from build123d import *

# Parameters (mm, degrees)
MODEL_R                 = 1.5
SALIENTE_EXTRUIR1_DEPTH = 3


with BuildPart() as part:
    # Model → Saliente-Extruir1 (new body)
    with BuildSketch(Plane.XY):
        with BuildLine():
            Line((149.34213351, 211.823953209), (158.34213351, 211.823953209))
            ThreePointArc((158.34213351, 211.823953209), (161.524114025, 210.505933724), (162.84213351, 207.323953209))
            Line((162.84213351, 207.323953209), (162.84213351, 193.823953209))
            Line((162.84213351, 193.823953209), (153.84213351, 193.823953209))
            Line((153.84213351, 193.823953209), (153.84213351, 202.823953209))
            Line((153.84213351, 202.823953209), (149.34213351, 202.823953209))
            ThreePointArc((149.34213351, 202.823953209), (144.84213351, 207.323953209), (149.34213351, 211.823953209))
        make_face()
        with Locations((149.34213351, 207.323953209)):
            Circle(MODEL_R, mode=Mode.SUBTRACT)
        with Locations((158.34213351, 207.323953209)):
            Circle(MODEL_R, mode=Mode.SUBTRACT)
        with BuildLine():
            Line((160.84213351, 196.698953209), (155.84213351, 196.698953209))
            ThreePointArc((155.84213351, 196.698953209), (155.311803424, 196.918623123), (155.09213351, 197.448953209))
            Line((155.09213351, 197.448953209), (155.09213351, 199.198953209))
            ThreePointArc((155.09213351, 199.198953209), (155.311803424, 199.729283295), (155.84213351, 199.948953209))
            Line((155.84213351, 199.948953209), (160.84213351, 199.948953209))
            ThreePointArc((160.84213351, 199.948953209), (161.372463595, 199.729283295), (161.59213351, 199.198953209))
            Line((161.59213351, 199.198953209), (161.59213351, 197.448953209))
            ThreePointArc((161.59213351, 197.448953209), (161.372463595, 196.918623123), (160.84213351, 196.698953209))
        make_face(mode=Mode.SUBTRACT)
    extrude(amount=SALIENTE_EXTRUIR1_DEPTH)


solid = part.part
Can you work these out from the model? Positions are in its coordinate system, mm. A direction names the side the tool comes from. Round coordinates to 2 decimals unless told otherwise and drop trailing zeros. Loops run counter-clockwise (first coordinate to the right, second up) from the corner with the lowest first, then second, coordinate; pieces in that order, holes last. Notation, with made-up numbers: (34, 20.5) - (75, 20.5) arc R16 cw to (75, 38.5) - close; hole circle Ø1 at (14.25, 7.25). An arc over 180 degrees is marked (long way). Answer in a Markdown table with one row per item. Add a question column.
Q1. For pin 1 Ø1 at (x, y) = (160.5, 204) entering from -Z; pin 2 Ø1.5 at (y, z) = (197.5, 1.5) entering from -X; pin 3 Ø2 at (x, y) = (151, 197.5) entering from +Z; pin 4 Ø0.9 at (x, z) = (152, 2) entering from -Y, each with a flat end and sliding along its axis, tell me the tip position at first contact or that it passes through.
Q2. I want a section at C-C on x = 159.5. List the corners of the cut face in (y, z) for me, and give its area (3 significant figures).
Q3. I want a section at A-A on x = 156.5. List the corners of the cut face in (y, z) for me.
Q4. I need wall thicknesses on L1, parallel to Y at x = 158.75, z = 2.25; L2, parallel to Y at x = 159.5, z = 1.2; L3, parallel to X at y = 206, z = 1. Which ranges of each line are inside material? Lowest first, please.
Q5. Which directions (+Z, -Z, +X, -X, +Y, -Y) give clear straight access to the entire face, cutting with the end or side of a thin tool? Please do faces 4 (the flat face through (152, 202.824, 1)), 5 (the flat face through (161.592, 198, 1)), 6 (the cylindrical face through (144.843, 207.225, 1.479)).
Q6. I want a section at B-B on z = 1. List the corners of the cut face in (x, y) for me.
Q7. I want a section at D-D on y = 201.25. List the corners of the cut face in (x, z) for me.
Q8. We'd pull the mould along X, two halves only. Please class faces 1 (the flat face through (155.092, 198, 1)), 2 (the flat face through (153.842, 198, 1)), 3 (the flat face through (158, 193.824, 1)): pulls with the +X half, pulls with the -X half, needs draft (parallel to the pull), parting line crosses it, or undercut.
A:
| question | item | result |
|---|---|---|
| 1 | pin 1 | z = 0 |
| 1 | pin 2 | x = 153.84 |
| 1 | pin 3 | through |
| 1 | pin 4 | y = 202.82 |
| 2 | outline | (193.82, 0) - (196.7, 0) - (196.7, 3) - (193.82, 3) - close; (199.95, 0) - (206.37, 0) - (206.37, 3) - (199.95, 3) - close; (208.28, 0) - (211.67, 0) - (211.67, 3) - (208.28, 3) - close |
| 2 | area | 38.1 mm^2 |
| 3 | outline | (193.82, 0) - (196.7, 0) - (196.7, 3) - (193.82, 3) - close; (199.95, 0) - (211.82, 0) - (211.82, 3) - (199.95, 3) - close |
| 4 | L1 | 193.82 to 196.7, 199.95 to 205.88, 208.77 to 211.81 |
| 4 | L2 | 193.82 to 196.7, 199.95 to 206.37, 208.28 to 211.67 |
| 4 | L3 | 145.04 to 148.64, 150.05 to 157.64, 159.05 to 162.84 |
| 5 | face 4 | +Z, -Z, -X, -Y |
| 5 | face 5 | +Z, -Z |
| 5 | face 6 | +Z, -Z, -X |
| 6 | outline | (149.34, 202.82) - (153.84, 202.82) - (153.84, 193.82) - (162.84, 193.82) - (162.84, 207.32) arc R4.5 ccw to (158.34, 211.82) - (149.34, 211.82) arc R4.5 ccw to start; hole circle Ø3 at (149.34, 207.32); hole (155.09, 197.45) arc R0.75 ccw to (155.84, 196.7) - (160.84, 196.7) arc R0.75 ccw to (161.59, 197.45) - (161.59, 199.2) arc R0.75 ccw to (160.84, 199.95) - (155.84, 199.95) arc R0.75 ccw to (155.09, 199.2) - close; hole circle Ø3 at (158.34, 207.32) |
| 7 | outline | (153.84, 0) - (162.84, 0) - (162.84, 3) - (153.84, 3) - close |
| 8 | face 1 | undercut |
| 8 | face 2 | pulls with the -X half |
| 8 | face 3 | needs draft |
